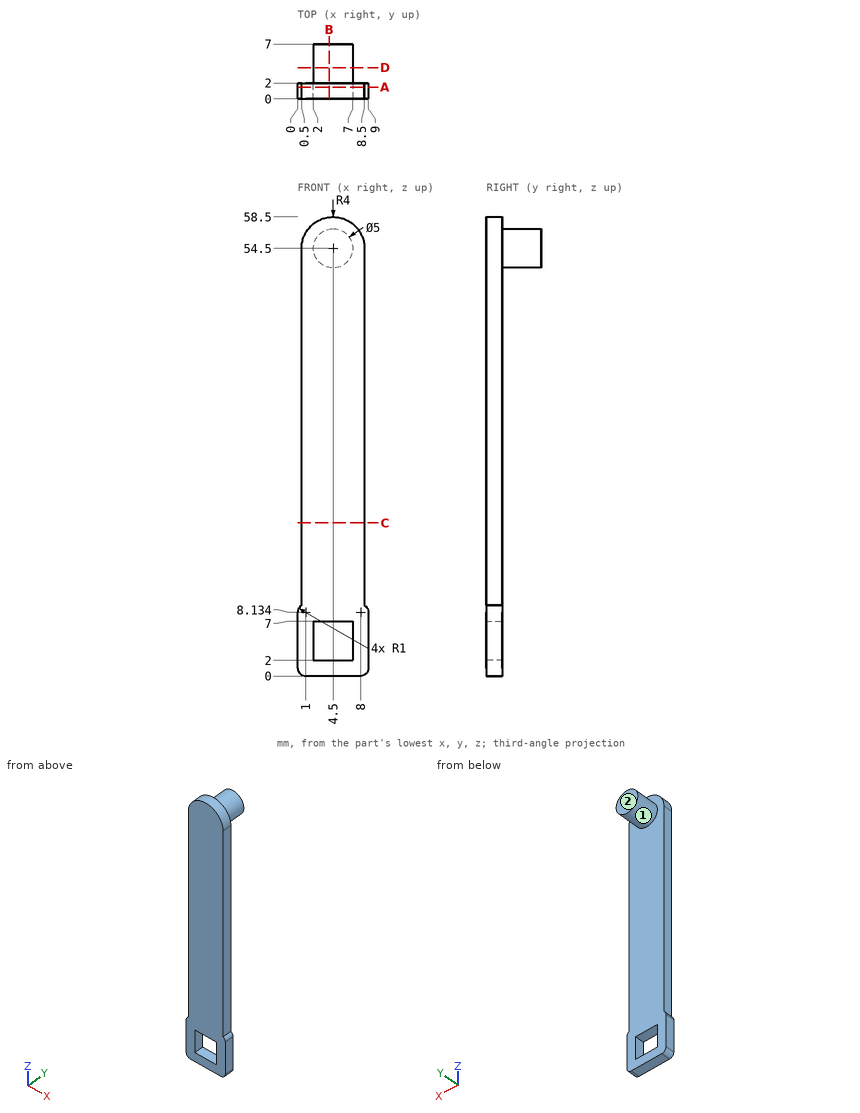
Input: dimensioned drawing with shaded views. Units: mm. Origin: part minimum x, y, z. A direction names the side the tool comes from. Coordinates: 2 decimals unless noted, no trailing zeros. Loops run counter-clockwise (first coordinate to the right, second up) from the corner with the lowest first, then second, coordinate; pieces in that order, holes last. Notation, with made-up numbers: (67, 20) -> (72, 20) arc R11 ccw to (72, 28) -> close; hole circle Ø8 at (52.5, 6). An arc over 180 degrees is marked (long way). Use a Markdown table: item, result. Add a question column.
(1) Line query: line 1 along Y through (x, z) = (8, 7.5); line 2 along X through (y, z) = (1.25, 26); line 3 along Z through (x, y) = (6.75, 6.75). Output: solid intervals per line, ascending.
(2) Section query D-D, the plane y = 4. Return loops of the section in (x, z).
(3) Section query B-B, the plane x = 4. Return loops of the section in (y, z).
(4) Section query A-A, the plane y = 1.5. Return loops of the section in (x, z).
(5) Pin query (flat end, axial travel): pin 1 Ø1.5 at (x, y) = (3, 1.5) entering from +Z; pin 2 Ø0.6 at (y, z) = (0.5, 41.5) entering from +X; pin 3 Ø1 at (y, z) = (1, 37) entering from -X. Return the tip coordinate at first contact, or that it passes through.
(6) Section query C-C, the plane z = 19.5. Return loops of the section in (x, y), plus the area to 3 significant figures.
(7) Access query for the marked faces 1 and 2. Directions: +Z, -Z, +X, -X, +Y, -Y. A direction counts if a zero-diameter tool reaches every point of the face in a straight line with its end or side. Return the directions, or none.
Answer:
| question | item | result |
|---|---|---|
| 1 | line 1 | y = 0 to 2 |
| 1 | line 2 | x = 0.5 to 8.5 |
| 1 | line 3 | z = 53.41 to 55.59 |
| 2 | outline | circle Ø5 at (4.5, 54.5) |
| 3 | outline | (0, 0) -> (2, 0) -> (2, 2) -> (0, 2) -> close; (0, 7) -> (2, 7) -> (2, 52.05) -> (7, 52.05) -> (7, 56.95) -> (2, 56.95) -> (2, 58.47) -> (0, 58.47) -> close |
| 4 | outline | (0, 1) arc R1 ccw to (1, 0) -> (8, 0) arc R1 ccw to (9, 1) -> (9, 8.13) arc R1 ccw to (8.5, 9) -> (8.5, 54.5) arc R4 ccw to (0.5, 54.5) -> (0.5, 9) arc R1 ccw to (0, 8.13) -> close; hole (2, 2) -> (7, 2) -> (7, 7) -> (2, 7) -> close |
| 5 | pin 1 | stops at z = 58.43 |
| 5 | pin 2 | stops at x = 8.5 |
| 5 | pin 3 | stops at x = 0.5 |
| 6 | outline | (0.5, 0) -> (8.5, 0) -> (8.5, 2) -> (0.5, 2) -> close |
| 6 | area | 16.0 mm^2 |
| 7 | face 1 | +Y |
| 7 | face 2 | +Z, -Z, +X, -X, +Y |
